Model file for the job. Use its own axes, mm. A direction names the side the tool comes from. Give positions to 0.01 mm unless a question says otherwise; leave off trailing zeros. Order: outer loops, then holes, each group sorted by start corner. A loop starts at its lowest first (then second) coordinate and runs counter-clockwise, first axis right, second up. Notation, with made-up numbers: (7, 61) -> (49, 61) arc R19 cw to (49, 72) -> close; hole circle Ø7 at (24.25, -15). An arc over 180 degrees is marked (long way). Use CSV: the item, a comma, the result in double quotes. Start each with the question number.
1. 3-axis set-ups, long thin cutter, end or side, ignore diameter. For faces 5 (the cylindrical face through (7.81, -28.02, -1.73)), 6 (the flat face through (5.2, -27.762, 0.1)): which of +Z, -Z, +X, -X, +Y, -Y reach the whole face in a straight line?
2. Cut at B-B on x = 0. List the corners of the cut face in (y, z), then the cut area to 3 significant figures.
3. Drop flat-ended pins along their axis: pin 1 (8 mm diameter, centred on x = -3.5, z = 3, fed in from +Y); pin 2 (2 mm diameter, centred on y = -16.5, z = -6, fed in from -X); pin 3 (1 mm diameter, centred on y = -10.5, z = -3.5, fed in from +X). Give the stop position or say it passes through.
4. Cut at D-D on y = -22.25. List the corners of the cut face in (x, z).
5. Cut at C-C on y = -12.25. List the corners of the cut face in (x, z), then the cut area to 3 significant figures.
6. Wall check: line 1 (Y direction, x = -5.5, z = -4.25); line 2 (X direction, y = -13.75, z = -4.25); line 3 (Z direction, x = 3.25, y = -21.25). Give the ranges that are in metal, low to high. Write a range as from..to.
7. Pull direction Y, two halves, no side cores. Call faces 1 (the conical face through (3.526, -21.545, -4.599)), 2 (the cylindrical face through (4.88, -29.78, -1.08)), 3 (the flat face through (0, -33.262, 0)), 4 (the cylindrical face through (-1.352, -25.269, 4.292)): released by +Y, released by -Y, zero draft, split by the parting line, or undercut.
8. Cut at A-A on z = 0. List the corners of the cut face in (x, y).
```python
from build123d import *


with BuildPart() as part:
    # Sketch1 → Revolve1 (revolve)
    with BuildSketch(Plane.XY, mode=Mode.PRIVATE) as revolve1_sk:
        with BuildLine():
            Line((0, -33.262039486), (0, -8.762039486))
            Line((0, -8.762039486), (-6.5, -8.762039486))
            ThreePointArc((-6.5, -8.762039486), (-8.986095711, -10.082953987), (-9.282911506, -12.88248741))
            Line((-9.282911506, -12.88248741), (-4.5, -24.762039486))
            Line((-4.5, -24.762039486), (-4.5, -25.762039486))
            Line((-4.5, -25.762039486), (-5, -25.762039486))
            Line((-5, -25.762039486), (-5, -27.762039486))
            Line((-5, -27.762039486), (-8, -27.762039486))
            Line((-8, -27.762039486), (-8, -28.262039486))
            Line((-8, -28.262039486), (-5, -28.262039486))
            Line((-5, -28.262039486), (-5, -31.262039486))
            Line((-5, -31.262039486), (-4, -32.262039486))
            Line((-4, -32.262039486), (-4, -33.262039486))
            Line((-4, -33.262039486), (0, -33.262039486))
        make_face()
        with BuildLine():
            Line((0, -8.762039486), (0, -7.998248901))
            ThreePointArc((0, -7.998248901), (-3.272360618, -8.189851173), (-6.5, -8.762039486))
            Line((-6.5, -8.762039486), (0, -8.762039486))
        make_face()
    revolve(revolve1_sk.sketch.rotate(Axis((0, 89.34036061, 0), (0, -1, 0)), 270), axis=Axis((0, 89.34036061, 0), (0, -1, 0)))


solid = part.part
```
Verdict:
1,face 5,"-Y"
1,face 6,"none"
2,outline,"(-33.26, -4) -> (-32.26, -4) -> (-31.26, -5) -> (-28.26, -5) -> (-28.26, -8) -> (-27.76, -8) -> (-27.76, -5) -> (-25.76, -5) -> (-25.76, -4.5) -> (-24.76, -4.5) -> (-12.88, -9.28) arc R3 ccw to (-8.76, -6.5) arc R28.04 ccw to (-8.76, 6.5) arc R3 ccw to (-12.88, 9.28) -> (-24.76, 4.5) -> (-25.76, 4.5) -> (-25.76, 5) -> (-27.76, 5) -> (-27.76, 8) -> (-28.26, 8) -> (-28.26, 5) -> (-31.26, 5) -> (-32.26, 4) -> (-33.26, 4) -> close"
2,area,"329 mm^2"
3,pin 1,"y = -8"
3,pin 2,"x = -6.17"
3,pin 3,"x = 8.81"
4,outline,"circle Ø11.02 at (0, 0)"
5,outline,"circle Ø18.92 at (0, 0)"
5,area,"281 mm^2"
6,line 1,"-28.26..-27.76, -18.68..-8.8"
6,line 2,"-7.86..7.86"
6,line 3,"-4.94..4.94"
7,face 1,"undercut"
7,face 2,"zero draft"
7,face 3,"released by -Y"
7,face 4,"undercut"
8,outline,"(-9.28, -12.88) -> (-4.5, -24.76) -> (-4.5, -25.76) -> (-5, -25.76) -> (-5, -27.76) -> (-8, -27.76) -> (-8, -28.26) -> (-5, -28.26) -> (-5, -31.26) -> (-4, -32.26) -> (-4, -33.26) -> (4, -33.26) -> (4, -32.26) -> (5, -31.26) -> (5, -28.26) -> (8, -28.26) -> (8, -27.76) -> (5, -27.76) -> (5, -25.76) -> (4.5, -25.76) -> (4.5, -24.76) -> (9.28, -12.88) arc R3 ccw to (6.5, -8.76) arc R28.04 ccw to (-6.5, -8.76) arc R3 ccw to start"
